The model under review builds one solid part; all positions refer to its coordinate system, in mm. Face numbers are marked on the shaded views. A direction names the side the tool comes from. Coordinates: 2 decimals unless noted, no trailing zeros. Write each loop counter-clockwise with the first axis right and the second up, starting at its lowest first coordinate (ties: lowest second). Pieces come first, ordered by that corner, then holes. Notation, with made-up numbers: (60.25, 42) - (69.25, 42) arc R24 cw to (69.25, 78) - close; hole circle Ø7 at (49.5, -4.75). An arc over 180 degrees is marked (long way). Put each result on its own line as item: value. Start each with the question number.
Item 1: For pin 1 (2.5 mm diameter, centred on x = 7, y = 1.5, fed in from -Z), flat-tipped, find the tip position at first contact; note if it passes through.
Item 2: Consider section D-D on x = 5.9. Give the boundary of the cut face in (y, z), then the cut area to 3 significant figures.
Item 3: To check wall thickness, follow L1, parallel to Y at x = 9.5, z = 11.5; L2, parallel to Y at x = 2.25, z = 4.5; L3, parallel to Z at x = 5.9, y = -2.5. State the ranges of each line that lie inside material, in increasing order. Write a range as [from, to].
Item 4: Consider section A-A on x = 10.5. Give the boundary of the cut face in (y, z).
Item 5: Machinability: for the marked faces 1 and 2, which of the approach directions +Z, -Z, +X, -X, +Y, -Y give a long, thin tool a straight path to every point of the face, cutting with its end or side? Answer none if there is none.
Item 6: Mouldability with a two-part tool opening along X and no side actions: class the marked faces 3, 4 and 5 as pulls with the +X half, pulls with the -X half, needs draft (parallel to the pull), parting line crosses it, or undercut.
Item 7: Consider section C-C on y = 2.75. Give the boundary of the cut face in (x, z).
Item 8: Consider section B-B on z = 7. Give the boundary of the cut face in (x, y).
```python
from build123d import *

# Parameters (mm, degrees)
F0_W     = 12
F0_H     = 14
F1_DEPTH = 3
F2_R     = 4.1
F3_DEPTH = 1
F4_W     = 12
F4_H     = 2
F5_DEPTH = 3
F6_W     = 12
F6_H     = 2
F6_H_2   = 12
F7_DEPTH = 3
F8_R     = 1


with BuildPart() as f1:
    # F0 (on Front) → F1 (new body)
    with BuildSketch(Plane.XZ):
        with Locations((6, 7)):
            Rectangle(F0_W, F0_H)
    extrude(amount=F1_DEPTH)

    # F2 (on face) → F3 (cut)
    with BuildSketch(Plane.XZ.offset(3)):
        with Locations((5.9, 6.09918)):
            Circle(F2_R)
    extrude(amount=-F3_DEPTH, mode=Mode.SUBTRACT)

    # F4 (on face) → F5 (join)
    with BuildSketch(Plane(origin=(0, 0, 0), x_dir=(-1, 0, 0), z_dir=(0, 1, 0))):
        with Locations((-6, 13)):
            Rectangle(F4_W, F4_H)
    extrude(amount=F5_DEPTH)

    # F6 (on face) → F7 (join)
    with BuildSketch(Plane(origin=(0, 3, 0), x_dir=(-1, 0, 0), z_dir=(0, 1, 0))):
        with Locations((-6, 13)):
            Rectangle(F6_W, F6_H)
        with Locations((-6, 6)):
            Rectangle(F6_W, F6_H_2)
    extrude(amount=F7_DEPTH)

    # F8
    f8_edges = [f1.edges().sort_by_distance(p)[0] for p in [
        (12, -3, 7),
        (0, -3, 7),
        (6, -3, 14),
        (6, -3, 0),
        (6, 6, 14),
        (0, 6, 7),
        (12, 6, 7),
        (6, 6, 0),
        (0, 1.5, 14),
        (12, 1.5, 14),
        (12, -1.5, 0),
        (12, 4.5, 0),
        (0, 4.5, 0),
        (0, -1.5, 0),
    ]]
    fillet(f8_edges, radius=F8_R)


solid = f1.part
```
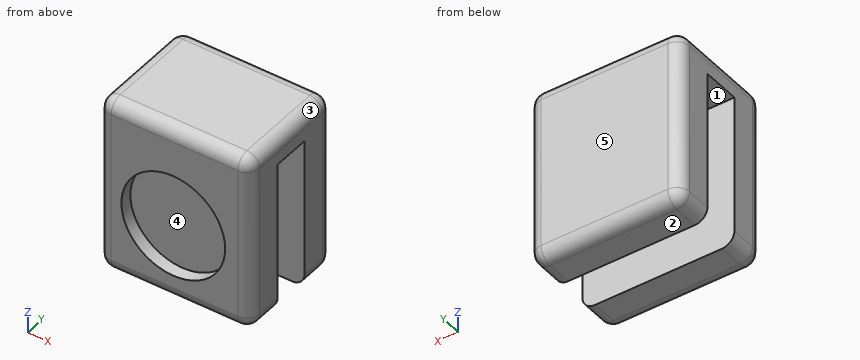
Report:
1. pin 1: z = 12
2. outline: (-3, 1) arc R1 ccw to (-2, 0) - (0, 0) - (0, 12) - (3, 12) - (3, 0) - (5, 0) arc R1 ccw to (6, 1) - (6, 13) arc R1 ccw to (5, 14) - (-2, 14) arc R1 ccw to (-3, 13) - (-3, 10.2) - (-2, 10.2) - (-2, 2) - (-3, 2) - close
2. area: 80.9 mm²
3. L1: [-3, 0], [3, 6]
3. L2: [-2, 0], [3, 6]
3. L3: [0.13, 2], [10.2, 13.87]
4. outline: (-3, 1) arc R1 ccw to (-2, 0) - (0, 0) - (0, 12) - (3, 12) - (3, 0) - (5, 0) arc R1 ccw to (6, 1) - (6, 13) arc R1 ccw to (5, 14) - (-2, 14) arc R1 ccw to (-3, 13) - close
5. face 1: -Z, +X, -X
5. face 2: -Z, +X, -X, +Y, -Y
6. face 3: pulls with the +X half
6. face 4: undercut
6. face 5: needs draft
7. outline: (0, 12) - (12, 12) - (12, 13) arc R1 ccw to (11, 14) - (1, 14) arc R1 ccw to (0, 13) - close
8. outline: (0, -2) arc R1 ccw to (1, -3) - (1.9, -3) - (1.9, -2) - (9.9, -2) - (9.9, -3) - (11, -3) arc R1 ccw to (12, -2) - (12, 0) - (0, 0) - close; (0, 3) - (12, 3) - (12, 5) arc R1 ccw to (11, 6) - (1, 6) arc R1 ccw to (0, 5) - close
